```python
from build123d import *

# Parameters (mm, degrees)
SKETCH1_W           = 731.52
SKETCH1_H           = 25.4
BOSS_EXTRUDE1_DEPTH = 50.8
SKETCH2_R           = 5.08
CUT_EXTRUDE1_DEPTH  = 53.34
SKETCH5_W           = 731.52
SKETCH5_H           = 40.64
CUT_EXTRUDE4_DEPTH  = 22.098


with BuildPart() as part:
    # Sketch1 → Boss-Extrude1 (new body)
    with BuildSketch(Plane(origin=(0, 0, 0), x_dir=(1, 0, 0), z_dir=(0, 1, 0))):
        with Locations((365.76, 12.7)):
            Rectangle(SKETCH1_W, SKETCH1_H)
    extrude(amount=BOSS_EXTRUDE1_DEPTH)

    # Sketch2 → Cut-Extrude1 (cut)
    with BuildSketch(Plane(origin=(0, 50.8, 0), x_dir=(1, 0, 0), z_dir=(0, 1, 0))):
        with Locations(Location((8.89, 12.7, 0), (0, 0, 270))):
            Circle(SKETCH2_R)
        with Locations(Location((22.86, 12.7, 0), (0, 0, 270))):
            Circle(SKETCH2_R)
        with Locations(Location((722.63, 12.7, 0), (0, 0, 270))):
            Circle(SKETCH2_R)
        with Locations(Location((708.66, 12.7, 0), (0, 0, 270))):
            Circle(SKETCH2_R)
    extrude(amount=-CUT_EXTRUDE1_DEPTH, mode=Mode.SUBTRACT)

    # Sketch5 → Cut-Extrude4 (cut)
    with BuildSketch(Plane.XY):
        with Locations((365.76, 25.4)):
            Rectangle(SKETCH5_W, SKETCH5_H)
    extrude(amount=-CUT_EXTRUDE4_DEPTH, mode=Mode.SUBTRACT)


solid = part.part
```
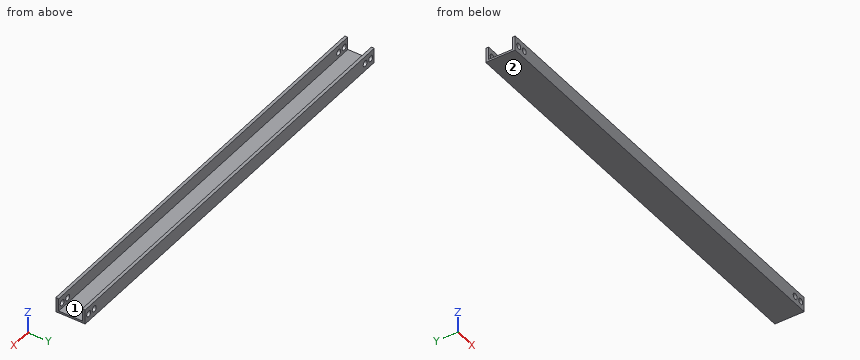
Input: part model. Units: mm. Frame: model coordinates. Face numbers are marked on the shaded views. A direction names the side the tool comes from. Coordinates: 2 decimals unless noted, no trailing zeros. Order: outer loops, then holes, each group sorted by start corner. A loop starts at its lowest first (then second) coordinate and runs counter-clockwise, first axis right, second up. Notation, with made-up numbers: (63, 4) - (70, 4) arc R10 ccw to (70, 17) - close; hole circle Ø5 at (-39, -5.75). An arc over 180 degrees is marked (long way). Return JSON: item names as keys, results as strings.
Q1. First-contact query: pin 1 (6 mm diameter, centred on x = 22.86, z = -12.7, fed in from +Y); pin 2 (5 mm diameter, centred on x = 615.5, y = 21.5, fed in from +Z). Flat tips, straight axial feed; report the tip coordinate or a pass-through.
The answers:
{"pin 1": "passes through", "pin 2": "stops at z = -22.1"}
Q2. Cut plane B-B (z = -12.7). State how many separate pieces and enclosed holes the cut face has, then the cut area to 3 significant figures.
The answers:
{"separate pieces": "10", "enclosed holes": "0", "area": "7,020 mm2"}
Q3. Cut plane C-C (y = 30). Return loops of the section in (x, z).
The answers:
{"outline": "(0, -25.4) - (731.52, -25.4) - (731.52, -22.1) - (0, -22.1) - close"}
Q4. Access query for the marked faces 1 and 2. Directions: +Z, -Z, +X, -X, +Y, -Y. A direction counts if a zero-diameter tool reaches every point of the face in a straight line with its end or side. Return the directions, or none.
The answers:
{"face 1": "+Z, +X, -X", "face 2": "-Z, +X, -X, +Y, -Y"}
Q5. Ray query, probe 1 along X at (y, z) = (3.5, -13.5); probe 2 along X at (y, z) = (49.55, -12.7); probe 3 along Y at (x, z) = (685, -17.25). Return the intervals inside material, ascending.
The answers:
{"probe 1": "x = 0 to 3.87, 13.91 to 17.84, 27.88 to 703.64, 713.68 to 717.61, 727.65 to 731.52", "probe 2": "x = 0 to 3.81, 13.97 to 17.78, 27.94 to 703.58, 713.74 to 717.55, 727.71 to 731.52", "probe 3": "y = 0 to 5.08, 45.72 to 50.8"}
Q6. Cut plane A-A (x = 676). Return loops of the section in (y, z), then the cut area to 3 significant figures.
The answers:
{"outline": "(0, -25.4) - (50.8, -25.4) - (50.8, 0) - (45.72, 0) - (45.72, -22.1) - (5.08, -22.1) - (5.08, 0) - (0, 0) - close", "area": "392 mm2"}
